```python
from build123d import *

# Parameters (mm, degrees)
SKETCH1_R               = 41.5925
BOSS_EXTRUDE1_DEPTH     = 165.1
CUT_EXTRUDE1_DEPTH      = 176.265176554
CUT_EXTRUDE1_DEPTH_BACK = 176.265176554
SKETCH2_R               = 12.7
SKETCH3_R               = 39.0525
CUT_EXTRUDE2_DEPTH      = 5.08
CUT_EXTRUDE3_START      = -2.54
SKETCH4_R               = 39.0525
SKETCH4_R_2             = 12.7
CUT_EXTRUDE3_DEPTH      = 2.54


with BuildPart() as part:
    # Sketch1 → Boss-Extrude1 (new body)
    with BuildSketch(Plane(origin=(0, 0, 0), x_dir=(1, 0, 0), z_dir=(0, 1, 0))):
        with Locations(Location((0, 0, 0), (0, 0, 270))):
            Circle(SKETCH1_R)
    extrude(amount=BOSS_EXTRUDE1_DEPTH)

    # Sketch2 → Cut-Extrude1 (cut, two sides: drawn at the far end of the back side and taken through both)
    with BuildSketch(Plane(origin=(0, 165.1, 0), x_dir=(1, 0, 0), z_dir=(0, 1, 0)).offset(-CUT_EXTRUDE1_DEPTH_BACK)):
        with Locations(Location((0, 0, 0), (0, 0, 270))):
            Circle(SKETCH2_R)
    extrude(amount=CUT_EXTRUDE1_DEPTH + CUT_EXTRUDE1_DEPTH_BACK, mode=Mode.SUBTRACT)

    # Sketch3 → Cut-Extrude2 (cut)
    with BuildSketch(Plane(origin=(0, 165.1, 0), x_dir=(1, 0, 0), z_dir=(0, 1, 0))):
        with Locations(Location((0, 0, 0), (0, 0, 270))):
            Circle(SKETCH3_R)
    extrude(amount=-CUT_EXTRUDE2_DEPTH, mode=Mode.SUBTRACT)

    # Sketch4 → Cut-Extrude3 (cut)
    with BuildSketch(Plane.XZ.offset(CUT_EXTRUDE3_START)):
        with Locations(Location((0, 0, 0), (0, 0, 90))):
            Circle(SKETCH4_R)
        with Locations(Location((0, 0, 0), (0, 0, 90))):
            Circle(SKETCH4_R_2, mode=Mode.SUBTRACT)
    extrude(amount=CUT_EXTRUDE3_DEPTH, mode=Mode.SUBTRACT)


solid = part.part
```
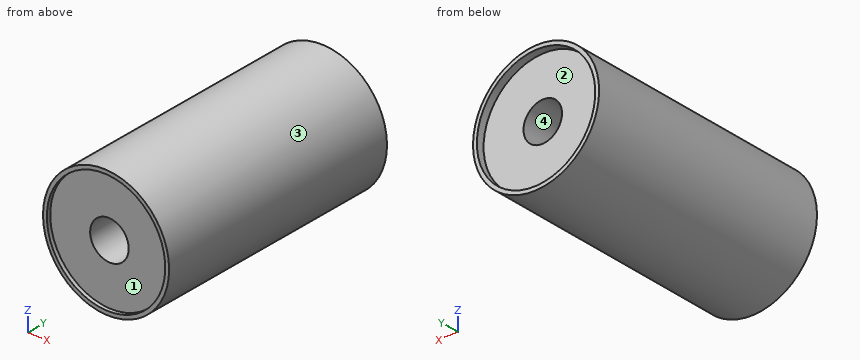
Verification items for the finished model (mm, model axes). Face numbers are marked on the shaded views. A direction names the side the tool comes from. Give positions to 0.01 mm unless a question says otherwise; leave off trailing zeros. Order: outer loops, then holes, each group sorted by start corner. A loop starts at its lowest first (then second) coordinate and runs counter-clockwise, first axis right, second up. Notation, with made-up numbers: (35, 55) -> (92, 55) arc R26 cw to (92, 79) -> close; hole circle Ø4 at (-27.75, 74). An arc over 180 degrees is marked (long way). One line per item, written item: value.
(1) Sectioned sample at B-B on z = 0. Record the cut outline in (x, y), then the cut area to 3 significant figures.
Final values:
outline: (-41.59, 0) -> (-39.05, 0) -> (-39.05, 2.54) -> (-12.7, 2.54) -> (-12.7, 160.02) -> (-39.05, 160.02) -> (-39.05, 165.1) -> (-41.59, 165.1) -> close; (12.7, 2.54) -> (39.05, 2.54) -> (39.05, 0) -> (41.59, 0) -> (41.59, 165.1) -> (39.05, 165.1) -> (39.05, 160.02) -> (12.7, 160.02) -> close
area: 9,140 mm^2
(2) Scan lines: line 1 along X through (y, z) = (120, 0); line 2 along X through (y, z) = (0.95, 0); line 3 along Y through (x, z) = (-7, 37). Record each from-to range of solid material in increasing order. Write a range as [from, to].
Final values:
line 1: [-41.59, -12.7], [12.7, 41.59]
line 2: [-41.59, -39.05], [39.05, 41.59]
line 3: [2.54, 160.02]
(3) Gauge pin test, flat ends, axial feed: pin 1 (10 mm diameter, centred on x = -14.5, z = -17, fed in from -Y); pin 2 (23.5 mm diameter, centred on x = 9.5, z = -2, fed in from +Y); pin 3 (1.5 mm diameter, centred on x = 31.5, y = 62.5, fed in from +Z). Record the tip position at first contact, or that the pin passes through.
Final values:
pin 1: y = 2.54
pin 2: y = 160.02
pin 3: z = 28.01
(4) Sectioned sample at D-D on z = 36. Record the cut outline in (x, y), then the cut area to 3 significant figures.
Final values:
outline: (-20.83, 0) -> (-15.14, 0) -> (-15.14, 2.54) -> (15.14, 2.54) -> (15.14, 0) -> (20.83, 0) -> (20.83, 165.1) -> (15.14, 165.1) -> (15.14, 160.02) -> (-15.14, 160.02) -> (-15.14, 165.1) -> (-20.83, 165.1) -> close
area: 6,650 mm^2
(5) Draft check along Z on the marked faces 3 and 4. Enter one of: pulls with the +Z half, pulls with the -Z half, needs draft (parallel to the pull), parting line crosses it, or undercut.
Final values:
face 3: parting line crosses it
face 4: undercut
(6) Sectioned sample at A-A on x = 0. Record the cut outline in (y, z), then the cut area to 3 significant figures.
Final values:
outline: (0, -41.59) -> (165.1, -41.59) -> (165.1, -39.05) -> (160.02, -39.05) -> (160.02, -12.7) -> (2.54, -12.7) -> (2.54, -39.05) -> (0, -39.05) -> close; (0, 39.05) -> (2.54, 39.05) -> (2.54, 12.7) -> (160.02, 12.7) -> (160.02, 39.05) -> (165.1, 39.05) -> (165.1, 41.59) -> (0, 41.59) -> close
area: 9,140 mm^2
(7) Tool access check on the marked faces 1 and 2. Record the directions out of +Z, -Z, +X, -X, +Y, -Y that give a thin tool (end or side, any length) a straight path to the whole face; none if there is none.
Final values:
face 1: -Y
face 2: +Y
(8) Sectioned sample at C-C on y = 33.5. Record the cut outline in (x, z) (1 decimal).
Final values:
outline: circle Ø83.2 at (0, 0); hole circle Ø25.4 at (0, 0)
